from build123d import *

# Parameters (mm, degrees)
SKETCH10_W          = 1
SKETCH10_H          = 30
BOSS_EXTRUDE1_DEPTH = 20
SKETCH11_R          = 2.6
CUT_EXTRUDE1_DEPTH  = 42.01792231
SKETCH12_R          = 7.5
CUT_EXTRUDE2_DEPTH  = 42.238966794


with BuildPart() as part:
    # Sketch10 → Boss-Extrude1 (new body)
    with BuildSketch(Plane.XY):
        with Locations((-17.929660394, 0.077000672)):
            Rectangle(SKETCH10_W, SKETCH10_H)
        with Locations((13.070339606, 0.077000672)):
            Rectangle(SKETCH10_W, SKETCH10_H)
        Polygon((-18.429660394, 16.077000672), (-18.429660394, 15.077000672), (-17.429660394, 15.077000672), (12.570339606, 15.077000672), (13.570339606, 15.077000672), (13.570339606, 16.077000672), align=None)
    extrude(amount=BOSS_EXTRUDE1_DEPTH)

    # Sketch11 → Cut-Extrude1 (cut, through all)
    with BuildSketch(Plane(origin=(13.570339606, 0, 0), x_dir=(0, 0, -1), z_dir=(1, 0, 0))):
        with Locations((-4.780263521, -5.922999328)):
            Circle(SKETCH11_R)
    extrude(amount=-CUT_EXTRUDE1_DEPTH, mode=Mode.SUBTRACT)

    # Sketch12 → Cut-Extrude2 (cut, through all)
    with BuildSketch(Plane(origin=(0, 16.077000672, 0), x_dir=(1, 0, 0), z_dir=(0, 1, 0))):
        with Locations(Location((-1.429660394, -10, 0), (0, 0, 270))):
            Circle(SKETCH12_R)
    extrude(amount=-CUT_EXTRUDE2_DEPTH, mode=Mode.SUBTRACT)


solid = part.part
Input: part model. Units: mm. Frame: model coordinates. A direction names the side the tool comes from. Coordinates: 2 decimals unless noted, no trailing zeros. Loops run counter-clockwise (first coordinate to the right, second up) from the corner with the lowest first, then second, coordinate; pieces in that order, holes last.
Q1. Cut plane C-C (x = 1). Output: boundary loops of the cut face in (y, z).
Q2. Cut plane D-D (y = -7). Output: boundary loops of the cut face in (x, z), then the cut area to 3 significant figures.
Q3. Contact query for a flat-ended pin moving along its axis: pin 1 (8.5 mm diameter, centred on y = -5.92, z = 4.78, fed in from -X). Output: stop coordinate, or through.
Q4. Set-up query: faces 4 (the face through (-1.1, 15.584, 2.507)), 5 (the face through (12.57, 0, 10)). Return all of +Z, -Z, +X, -X, +Y, -Y with unobstructed straight access to the full face (end or side cutting, diameter ignored); none if empty.
Q5. Material intervals for line 1 (X direction, y = 15.85, z = 10); line 2 (X direction, y = -9, z = 2.25); line 3 (Y direction, x = -11.5, z = 4.5), sorted ascending.
Q6. Cut plane A-A (y = 2). Output: boundary loops of the cut face in (x, z).
Q7. Cut plane B-B (z = 10). Output: boundary loops of the cut face in (x, y).
Q8. Draft query along Z for faces 1 (the face through (13, -14.923, 10)), 2 (the face through (-17.923, -5.809, 7.378)), 3 (the face through (-2.5, 15.6, 0)). Return one class per face: +Z half, -Z half, draft (parallel to the pull), parting line (faces both ways), or undercut.
Working result:
1. outline: (15.08, 0) - (16.08, 0) - (16.08, 2.9) - (15.08, 2.9) - close; (15.08, 17.1) - (16.08, 17.1) - (16.08, 20) - (15.08, 20) - close
2. outline: (-18.43, 0) - (-17.43, 0) - (-17.43, 2.41) - (-18.43, 2.41) - close; (-18.43, 7.15) - (-17.43, 7.15) - (-17.43, 20) - (-18.43, 20) - close; (12.57, 0) - (13.57, 0) - (13.57, 2.41) - (12.57, 2.41) - close; (12.57, 7.15) - (13.57, 7.15) - (13.57, 20) - (12.57, 20) - close
2. area: 30.5 mm2
3. pin 1: stops at x = -18.43
4. face 4: +Y, -Y
4. face 5: +Z, -Z, -Y
5. line 1: x = -18.43 to -8.93, 6.07 to 13.57
5. line 2: x = -18.43 to -17.43, 12.57 to 13.57
5. line 3: y = 15.08 to 16.08
6. outline: (-18.43, 0) - (-17.43, 0) - (-17.43, 20) - (-18.43, 20) - close; (12.57, 0) - (13.57, 0) - (13.57, 20) - (12.57, 20) - close
7. outline: (-18.43, -14.92) - (-17.43, -14.92) - (-17.43, 15.08) - (-8.93, 15.08) - (-8.93, 16.08) - (-18.43, 16.08) - close; (6.07, 15.08) - (12.57, 15.08) - (12.57, -14.92) - (13.57, -14.92) - (13.57, 16.08) - (6.07, 16.08) - close
8. face 1: draft
8. face 2: undercut
8. face 3: -Z half
